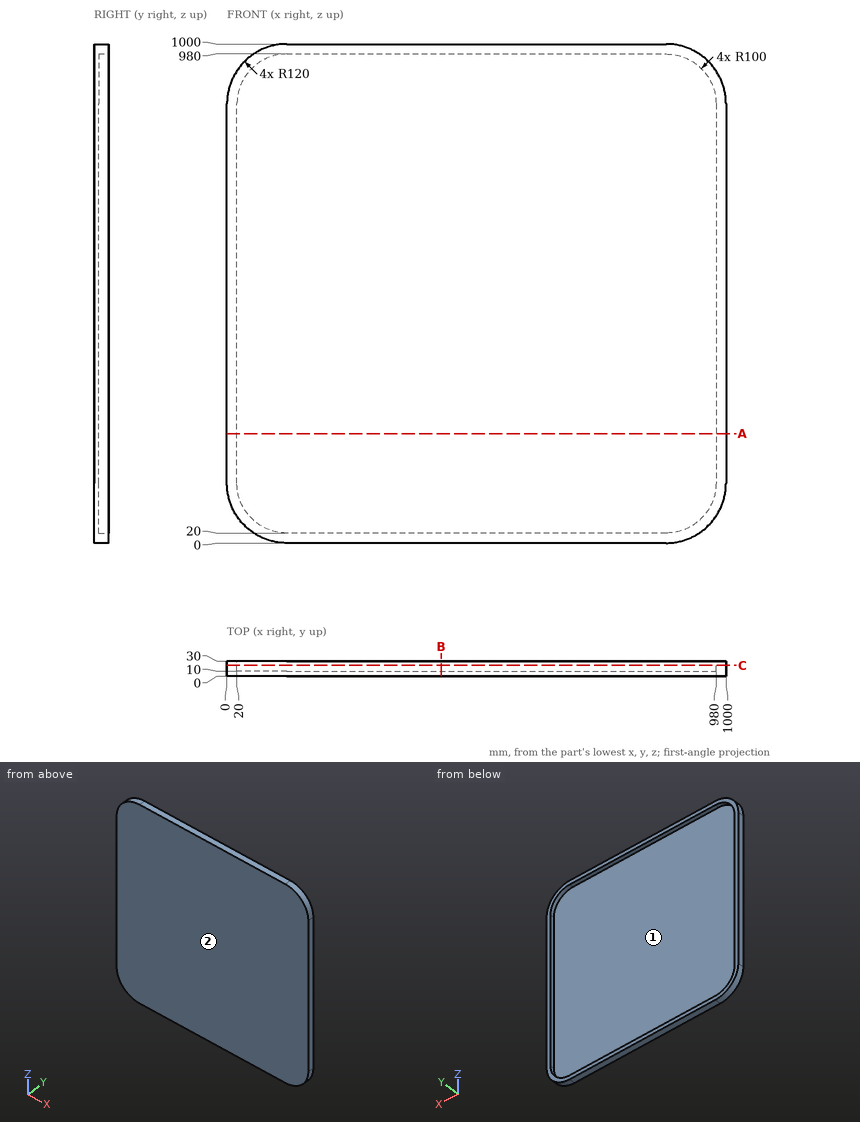
Geometry check sheet. Reference: drawing and pictorial views, mm from the part's lowest x, y, z. Coordinates: 2 decimals unless noted, no trailing zeros. Order: outer loops, then holes, each group sorted by start corner. A loop starts at its lowest first (then second) coordinate and runs counter-clockwise, first axis right, second up. Notation, with made-up numbers: (-39, 75.25) -> (-17, 75.25) arc R35 cw to (-17, 114.25) -> close; hole circle Ø2 at (-13.75, -21.75). An arc over 180 degrees is marked (long way). Use CSV: the item, a comma, the result in double quotes. Start each with the question number.
Q1. Depth check by flat-ended pin: P1, Ø2, axis at y = 16.5, z = 101.5, coming from the +X side; P2, Ø12, axis at x = 594, z = 255.5, coming from the +Y side. Enter the tip coordinate at first touch or a pass-through.
Q2. Draft check along Z on the marked faces 1 and 2. Enter one of: +Z half, -Z half, draft (parallel to the pull), parting line (faces both ways), or undercut.
Q3. Section check A-A, the plane z = 219. Record the cut outline in (x, y), and give its area (3 significant figures).
Q4. Section check C-C, the plane y = 21.5. Record the cut outline in (x, z), and give its area (3 significant figures).
Q5. Section check B-B, the plane x = 429. Record the cut outline in (y, z), and give its area (3 significant figures).
Q6. Thickness scan on line 1 along Z through (x, y) = (849.5, 21.25); line 2 along Y through (x, z) = (236.5, 951). Record the ranges inside material, lowest first.
Returned:
1,P1,"stops at x = 998.72"
1,P2,"stops at y = 10"
2,face 1,"undercut"
2,face 2,"draft"
3,outline,"(0, 0) -> (1000, 0) -> (1000, 30) -> (980, 30) -> (980, 10) -> (20, 10) -> (20, 30) -> (0, 30) -> close"
3,area,"10,800 mm^2"
4,outline,"(0, 120) arc R120 ccw to (120, 0) -> (880, 0) arc R120 ccw to (1000, 120) -> (1000, 880) arc R120 ccw to (880, 1000) -> (120, 1000) arc R120 ccw to (0, 880) -> close; hole (20, 120) arc R100 ccw to (120, 20) -> (880, 20) arc R100 ccw to (980, 120) -> (980, 880) arc R100 ccw to (880, 980) -> (120, 980) arc R100 ccw to (20, 880) -> close"
4,area,"74,600 mm^2"
5,outline,"(0, 0) -> (30, 0) -> (30, 20) -> (10, 20) -> (10, 980) -> (30, 980) -> (30, 1000) -> (0, 1000) -> close"
5,area,"10,800 mm^2"
6,line 1,"z = 0 to 20, 980 to 1000"
6,line 2,"y = 0 to 10"
